from build123d import *

# Parameters (mm, degrees)
BOX004_W     = 4
BOX004_H     = 11
BOX004_DEPTH = 2
BOX002_W     = 10
BOX002_H     = 13
BOX002_DEPTH = 6
BOX001_W     = 13
BOX001_H     = 7
BOX001_DEPTH = 6
PAD003_DEPTH = 4
SKETCH002_W  = 40
SKETCH002_H  = 16.5
SKETCH002_R  = 1.75
PAD002_DEPTH = 2
BOX003_W     = 13
BOX003_H     = 5
BOX003_DEPTH = 2


with BuildPart() as cube004:
    # Box004 → Box004 (new body)
    with BuildSketch(Plane(origin=(24, 0, -2), x_dir=(1, 0, 0), z_dir=(0, 0, 1))):
        with Locations((2, 5.5)):
            Rectangle(BOX004_W, BOX004_H)
    extrude(amount=BOX004_DEPTH)


with BuildPart() as cube002:
    # Box002 → Box002 (new body)
    with BuildSketch(Plane(origin=(26, -1, 2), x_dir=(1, 0, 0), z_dir=(0, 0, 1))):
        with Locations((5, 6.5)):
            Rectangle(BOX002_W, BOX002_H)
    extrude(amount=BOX002_DEPTH)


with BuildPart() as cube001:
    # Box001 → Box001 (new body)
    with BuildSketch(Plane(origin=(3, -2, 2), x_dir=(1, 0, 0), z_dir=(0, 0, 1))):
        with Locations((6.5, 3.5)):
            Rectangle(BOX001_W, BOX001_H)
    extrude(amount=BOX001_DEPTH)


with BuildPart() as fusion005:
    # Sketch003 → Pad003 (new body)
    with BuildSketch(Plane.XY.offset(3)):
        Polygon((15.32428, -1.087794), (15.32428, -2.777316), (2.472262, -4.853757), (1.271945, -5.617596), (-0.446694, -5.153837), (-0.228454, -4.717358), (1.080985, -5.071997), (2.335863, -4.308158), (14.655511, -2.390134), (14.655511, -1.087794), align=None)
    extrude(amount=PAD003_DEPTH)

    # Fusion005: union Cube001
    add(cube001.part)


with BuildPart() as pad002:
    # Sketch002 → Pad002 (new body)
    with BuildSketch(Plane.XY):
        with Locations((17, 5.25)):
            Rectangle(SKETCH002_W, SKETCH002_H)
        Circle(SKETCH002_R, mode=Mode.SUBTRACT)
        with Locations((19, 0)):
            Circle(SKETCH002_R, mode=Mode.SUBTRACT)
    extrude(amount=PAD002_DEPTH)


with BuildPart() as endstop:
    # Box003 → Box003 (new body)
    with BuildSketch(Plane(origin=(3, 4, -2), x_dir=(1, 0, 0), z_dir=(0, 0, 1))):
        with Locations((6.5, 2.5)):
            Rectangle(BOX003_W, BOX003_H)
    extrude(amount=BOX003_DEPTH)

    # Fusion006: union Cube004, Cube002, Fusion005, Pad002
    add(cube004.part)
    add(cube002.part)
    add(fusion005.part)
    add(pad002.part)


solid = endstop.part
The listing builds one solid part. Answer for the finished solid, in the listing's coordinates (mm). A direction names the side the tool comes from. Give positions to 0.01 mm unless a question says otherwise; leave off trailing zeros. Order: outer loops, then holes, each group sorted by start corner. A loop starts at its lowest first (then second) coordinate and runs counter-clockwise, first axis right, second up. Notation, with made-up numbers: (29, 48) - (72, 48) arc R22 cw to (72, 81) - close; hole circle Ø10 at (-20, 79). An arc over 180 degrees is marked (long way). Answer as CSV lines item,"result".
Q1. Which of the six approach directions +Z, -Z, +X, -X, +Y, -Y give full straight-line access (tool end or side, diameter ignored) to faces 1 (the face through (8.409, -3.363, 4.972)), 2 (the face through (9, 4, -1)), 3 (the face through (36, 5, 5)), 4 (the face through (26, 0, -1)), 5 (the face through (3, 1, 5))?
Answer key:
face 1,"+Z, -X"
face 2,"-Z, -X, -Y"
face 3,"+Z, +X, +Y, -Y"
face 4,"-Z, +X, -X, -Y"
face 5,"+Z, -X, +Y"
Q2. A cutting plane is placed at B-B, the plane z = 6.5. Determine the outline of the cut face in (x, y).
Answer key:
outline,"(-0.45, -5.15) - (1.27, -5.62) - (2.47, -4.85) - (15.32, -2.78) - (15.32, -2) - (16, -2) - (16, 5) - (3, 5) - (3, -2) - (14.66, -2) - (14.66, -2.39) - (2.34, -4.31) - (1.08, -5.07) - (-0.23, -4.72) - close; (26, -1) - (36, -1) - (36, 12) - (26, 12) - close"
Q3. A cutting plane is placed at C-C, the plane z = 0.5. Determine the outline of the cut face in (x, y), and give its area (3 significant figures).
Answer key:
outline,"(-3, -3) - (37, -3) - (37, 13.5) - (-3, 13.5) - close; hole circle Ø3.5 at (0, 0); hole circle Ø3.5 at (19, 0)"
area,"641 mm^2"
Q4. A cutting plane is placed at D-D, the plane y = 3.5. Determine the outline of the cut face in (x, z).
Answer key:
outline,"(-3, 0) - (24, 0) - (24, -2) - (28, -2) - (28, 0) - (37, 0) - (37, 2) - (36, 2) - (36, 8) - (26, 8) - (26, 2) - (16, 2) - (16, 8) - (3, 8) - (3, 2) - (-3, 2) - close"
Q5. Each of these flat-tipped pins is pushed along its axis until it touches: pin 1 Ø3 at (y, z) = (1, 4.5) entering from +X; pin 2 Ø5 at (x, z) = (12.5, 5.5) entering from -Y; pin 3 Ø5 at (x, z) = (21.5, 0) entering from -Y. Where does it stop, or does it pass through?
Answer key:
pin 1,"stops at x = 36"
pin 2,"stops at y = -3.64"
pin 3,"stops at y = -3"
Q6. Determine the mould class of faces 6 (the face through (26, 5, 5)), 7 (the face through (9, 2, 8)), 8 (the face through (9, -3.8, 5)) for opening direction X: pulls with the +X half, pulls with the -X half, needs draft (parallel to the pull), parting line crosses it, or undercut.
Answer key:
face 6,"undercut"
face 7,"needs draft"
face 8,"pulls with the +X half"
Q7. A cutting plane is placed at A-A, the plane x = 19. Determine the outline of the cut face in (y, z), and give its area (3 significant figures).
Answer key:
outline,"(-3, 0) - (-1.75, 0) - (-1.75, 2) - (-3, 2) - close; (1.75, 0) - (13.5, 0) - (13.5, 2) - (1.75, 2) - close"
area,"26.0 mm^2"
Q8. Straight lines are drawn through the part: L1, parallel to X at y = 2.5, z = 3.5; L2, parallel to Y at x = 19, z = 1; L3, parallel to Z at x = 33, y = 11.5. For each, find the intervals that lie inside material, in ascending order.
Answer key:
L1,"x = 3 to 16, 26 to 36"
L2,"y = -3 to -1.75, 1.75 to 13.5"
L3,"z = 0 to 8"
